For this review, take the finished solid that the model builds, in its own axes (mm). Give positions to 0.01 mm unless a question says otherwise; leave off trailing zeros. Loops run counter-clockwise (first coordinate to the right, second up) from the corner with the lowest first, then second, coordinate; pieces in that order, holes last. Notation, with made-up numbers: (-38.75, -32) - (-24.75, -32) arc R16 cw to (-24.75, -20) - close; hole circle Ø10 at (4.25, 78.5). An arc over 180 degrees is marked (long way). Use CSV: the item, a comma, the result in double quotes. Start each with the question number.
1. Take a section at A-A on x = 100. Give the boundary of the cut face in (y, z).
2. Take a section at B-B on x = 73. Give the boundary of the cut face in (y, z).
3. Wall thickness on line 1 (X direction, y = 22, z = -19); line 2 (Y direction, x = 25, z = -43.5); line 3 (Z direction, x = 100, y = 17.25): over which ranges is each line inside the solid? List them lowest first.
4. For pin 1 (1.5 mm diameter, centred on x = 69, z = -20.5, fed in from +Y); pin 2 (6 mm diameter, centred on x = 87.59, z = -17.18, fed in from +Y), all flat-tipped, find the tip position at first contact; note any pin that passes through.
5. Take a section at C-C on x = 54. Give the boundary of the cut face in (y, z).
```python
from build123d import *

# Parameters (mm, degrees)
SKETCH1_W                       = 152.4
SKETCH1_H                       = 95.25
BOSS_EXTRUDE1_DEPTH             = 25.4
SKETCH2_R                       = 38.1
F_3IN_POCKET_DEPTH              = 2.54
CLAMP_POCKET_DEPTH              = 4.7498
SKETCH4_R                       = 1.89865
NO25_THREAD_FORM_FOR_8_32_DEPTH = 20.6502
FOUR_CLAMPS_COUNT               = 4
F_180_CLAMP_COUNT               = 2
F_180_CLAMP_ANGLE               = 135
F_360_CLAMP_COUNT               = 2
F_360_CLAMP_ANGLE               = 315


with BuildPart() as part:
    # Sketch1 → Boss-Extrude1 (new body)
    with BuildSketch(Plane(origin=(0, 0, 0), x_dir=(1, 0, 0), z_dir=(0, 1, 0))):
        with Locations((76.2, 47.625)):
            Rectangle(SKETCH1_W, SKETCH1_H)
    extrude(amount=BOSS_EXTRUDE1_DEPTH)

    # Sketch2 → 3in Pocket (cut)
    with BuildSketch(Plane(origin=(0, 25.4, 0), x_dir=(1, 0, 0), z_dir=(0, 1, 0))):
        with Locations((57.15, 47.625)):
            Circle(SKETCH2_R)
    extrude(amount=-F_3IN_POCKET_DEPTH, mode=Mode.SUBTRACT)

    # Sketch3 → Clamp Pocket (cut)
    with BuildSketch(Plane(origin=(0, 25.4, 0), x_dir=(1, 0, 0), z_dir=(0, 1, 0))):
        with BuildLine():
            Line((90.736157893, 67.740773711), (97.471349984, 74.475965802))
            ThreePointArc((97.471349984, 74.475965802), (98.401285953, 76.721029832), (97.471349984, 78.966093863))
            Line((97.471349984, 78.966093863), (88.491093863, 87.946349984))
            ThreePointArc((88.491093863, 87.946349984), (86.246029832, 88.876285953), (84.000965802, 87.946349984))
            Line((84.000965802, 87.946349984), (77.265773711, 81.211157893))
            ThreePointArc((77.265773711, 81.211157893), (76.335837741, 78.966093863), (77.265773711, 76.721029832))
            Line((77.265773711, 76.721029832), (86.246029832, 67.740773711))
            ThreePointArc((86.246029832, 67.740773711), (88.491093863, 66.810837741), (90.736157893, 67.740773711))
        make_face()
    clamp_pocket = extrude(amount=-CLAMP_POCKET_DEPTH, mode=Mode.SUBTRACT)

    # Sketch4 → No25 Thread Form for 8-32 (cut)
    with BuildSketch(Plane(origin=(0, 20.6502, 0), x_dir=(1, 0, 0), z_dir=(0, 1, 0))):
        with Locations((87.59306825, 78.06806825)):
            Circle(SKETCH4_R)
    no25_thread_form_for_8_32 = extrude(amount=-NO25_THREAD_FORM_FOR_8_32_DEPTH, mode=Mode.SUBTRACT)

    # Four Clamps: Clamp Pocket, No25 Thread Form for 8-32 ×4 about axis
    four_clamps_axis = Axis((57.15, 0, -47.625), (0, 1, 0))
    for i in range(1, FOUR_CLAMPS_COUNT):
        add(clamp_pocket.rotate(four_clamps_axis, i * 360 / FOUR_CLAMPS_COUNT), mode=Mode.SUBTRACT)
        add(no25_thread_form_for_8_32.rotate(four_clamps_axis, i * 360 / FOUR_CLAMPS_COUNT), mode=Mode.SUBTRACT)

    # 180 Clamp: Clamp Pocket, No25 Thread Form for 8-32 ×2 about axis
    f_180_clamp_axis = Axis((57.15, 0, -47.625), (0, 1, 0))
    for i in range(1, F_180_CLAMP_COUNT):
        add(clamp_pocket.rotate(f_180_clamp_axis, i * F_180_CLAMP_ANGLE / (F_180_CLAMP_COUNT - 1)), mode=Mode.SUBTRACT)
        add(no25_thread_form_for_8_32.rotate(f_180_clamp_axis, i * F_180_CLAMP_ANGLE / (F_180_CLAMP_COUNT - 1)), mode=Mode.SUBTRACT)

    # 360 Clamp: Clamp Pocket, No25 Thread Form for 8-32 ×2 about axis
    f_360_clamp_axis = Axis((57.15, 25.4, -47.625), (0, 1, 0))
    for i in range(1, F_360_CLAMP_COUNT):
        add(clamp_pocket.rotate(f_360_clamp_axis, i * F_360_CLAMP_ANGLE / (F_360_CLAMP_COUNT - 1)), mode=Mode.SUBTRACT)
        add(no25_thread_form_for_8_32.rotate(f_360_clamp_axis, i * F_360_CLAMP_ANGLE / (F_360_CLAMP_COUNT - 1)), mode=Mode.SUBTRACT)


solid = part.part
```
Check result:
1,outline,"(0, -95.25) - (25.4, -95.25) - (25.4, -57.15) - (20.65, -57.15) - (20.65, -49.51) - (0, -49.51) - close; (0, -45.74) - (20.65, -45.74) - (20.65, -38.1) - (25.4, -38.1) - (25.4, 0) - (0, 0) - close"
2,outline,"(0, -95.25) - (25.4, -95.25) - (25.4, -82.27) - (22.86, -82.27) - (22.86, -12.98) - (25.4, -12.98) - (25.4, 0) - (0, 0) - close"
3,line 1,"x = 0 to 15.93, 36.56 to 77.74, 98.37 to 152.4"
3,line 2,"y = 0 to 22.86"
3,line 3,"z = -95.25 to -49.51, -45.74 to 0"
4,pin 1,"stops at y = 22.86"
4,pin 2,"stops at y = 20.65"
5,outline,"(0, -95.25) - (25.4, -95.25) - (25.4, -85.59) - (22.86, -85.59) - (22.86, -9.66) - (25.4, -9.66) - (25.4, 0) - (0, 0) - close"
